Geometry: final body of the model. Coordinates: model frame, mm. Face numbers are marked on the shaded views. A direction names the side the tool comes from. Give positions to 0.01 mm unless a question says otherwise; leave off trailing zeros. Write each loop counter-clockwise with the first axis right and the second up, starting at its lowest first coordinate (ties: lowest second). Pieces come first, ordered by that corner, then holes.
Q1. Reachability of the marked faces 1, 2, 3, 4 and 5 from +Z, -Z, +X, -X, +Y, -Y: full face, straight path, thin tool, end or side. Return the list, or none.
Q2. Cut plane A-A on y = 4. Count the separate pieces of the cut face and the enclosed holes in it, plus the area to 3 significant figures.
Q3. Cut plane B-B on z = 22. Return the cut outline in (x, y).
Q4. Pin query (flat end, axial travel): pin 1 (1.5 mm diameter, centred on x = 19, z = 86, fed in from -Y); pin 2 (1 mm diameter, centred on x = 5, z = 21, fed in from -Y); pin 3 (2 mm diameter, centred on x = 15.5, y = 1, fed in from -Z); pin 4 (1.5 mm diameter, centred on x = 37, y = 48, fed in from -Z). Return the tip coordinate at first contact, or that it passes through.
Q5. Line query: L1, parallel to Y at x = 42.5, z = 86.45; L2, parallel to X at y = 30.5, z = 11; L3, parallel to Z at x = -9.5, y = 29.5. Output: solid intervals per line, ascending.
```python
from build123d import *

# Parameters (mm, degrees)
F1_DEPTH = 60
F3_R     = 1.75
F3_W     = 3.5
F3_H     = 8
F3_W_2   = 2
F3_W_3   = 33
F4_DEPTH = 3
F6_W     = 37
F6_H     = 35
F5_W     = 60
F5_H     = 60
F10_W    = 56
F10_H    = 56


# Not quite as in the source:
# - a feature names something its author has since deleted; it is built from what else it names


with BuildPart() as f1:
    # F0 (on Top) → F1 (new body)
    with BuildSketch(Plane.XY):
        Polygon((-2, 0), (0, 0), (0, 33), (33, 33), (33, 0), (35, 0), (35, 35), (-2, 35), align=None)
    extrude(amount=F1_DEPTH)



with BuildPart() as f4:
    # F3 (on offset) → F4 (new body)
    with BuildSketch(Plane.XY.offset(85)):
        Polygon((-13.5, 0), (-5.5, 0), (-5.5, 8), (-5.5, 52), (38.5, 52), (38.5, 8), (38.5, 0), (46.5, 0), (46.5, 60), (-13.5, 60), align=None)
        with Locations((-9.5, 4)):
            Circle(F3_R, mode=Mode.SUBTRACT)
        with Locations((42.5, 4)):
            Circle(F3_R, mode=Mode.SUBTRACT)
        with Locations((-9.5, 56)):
            Circle(F3_R, mode=Mode.SUBTRACT)
        with Locations((42.5, 56)):
            Circle(F3_R, mode=Mode.SUBTRACT)
        with Locations((-3.75, 4)):
            Rectangle(F3_W, F3_H)
        with Locations((36.75, 4)):
            Rectangle(F3_W, F3_H)
        with Locations((34, 4)):
            Rectangle(F3_W_2, F3_H)
        with Locations((-1, 4)):
            Rectangle(F3_W_2, F3_H)
        with Locations((16.5, 4)):
            Rectangle(F3_W_3, F3_H)
    extrude(amount=F4_DEPTH)


with BuildPart() as f1_1:
    add(f1.part)

    add(f4.part)  # F7 merges F4
    # F6 (on face) → F7 section 0
    with BuildSketch(Plane.XY.offset(60)):
        with Locations((16.5, 17.5)):
            Rectangle(F6_W, F6_H)
    # F5 (on face) → F7 section 1
    with BuildSketch(Plane.XY.offset(85)):
        with Locations((16.5, 30)):
            Rectangle(F5_W, F5_H)
    loft()


with BuildPart() as f11:
    # F10 (on offset) → F11 section 0
    with BuildSketch(Plane(origin=(0, 0, 85), x_dir=(1, 0, 0), z_dir=(0, 0, -1))):
        with Locations((16.5, -30)):
            Rectangle(F10_W, F10_H)
    # F9 (on face) → F11 section 1
    with BuildSketch(Plane.XY.offset(60)):
        Polygon((0, 33), (0, 2), (2, 2), (4, 2), (29, 2), (31, 2), (33, 2), (33, 33), align=None)
    loft()


with BuildPart() as f1_2:
    add(f1_1.part)

    # F13: cut F11
    add(f11.part, mode=Mode.SUBTRACT)


solid = f1_2.part
```
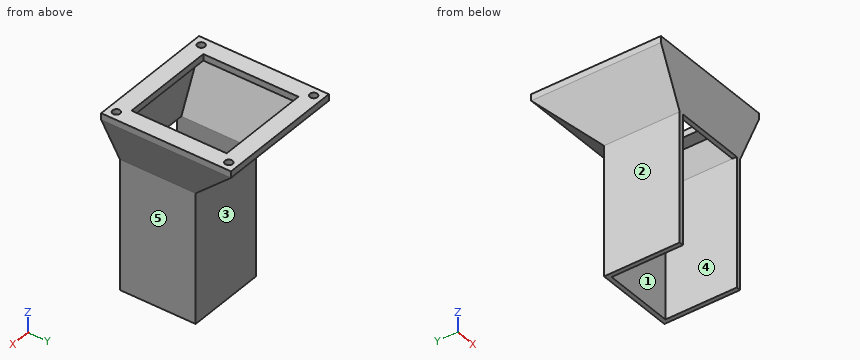
Data:
1. face 1: +Z, -Z, -Y
1. face 2: -Z, -X, +Y, -Y
1. face 3: -Z, +X, -X, +Y
1. face 4: -Z, -Y
1. face 5: -Z, +X, +Y, -Y
2. separate pieces: 3
2. enclosed holes: 0
2. area: 499 mm2
3. outline: (-2, 0) - (0, 0) - (0, 33) - (33, 33) - (33, 0) - (35, 0) - (35, 35) - (-2, 35) - close
4. pin 1: stops at y = 0
4. pin 2: stops at y = 33
4. pin 3: stops at z = 60
4. pin 4: stops at z = 72.25
5. L1: y = 0 to 2.25, 5.75 to 54.25, 57.75 to 60
5. L2: x = -2 to 0, 33 to 35
5. L3: z = 76.3 to 80.65, 85 to 88
